For this review, take the finished solid that the model builds, in its own axes (mm). A direction names the side the tool comes from. Round coordinates to 2 decimals unless told otherwise and drop trailing zeros. Order: outer loops, then holes, each group sorted by start corner. A loop starts at its lowest first (then second) coordinate and runs counter-clockwise, first axis right, second up. Notation, with made-up numbers: (-40, 89.5) - (16, 89.5) arc R14 cw to (16, 101.5) - close; hole circle Ø4 at (53.25, 55). An arc over 180 degrees is marked (long way). One line per question, with ' | ' between items.
```python
from build123d import *

# Parameters (mm, degrees)
F0_W     = 480
F0_H     = 190
F1_DEPTH = 20
F2_W     = 500
F2_H     = 300
F3_DEPTH = 20
F4_W     = 10
F4_H     = 20
F4_W_2   = 500
F5_DEPTH = 170


# Not quite as in the source:
# - the program builds the solid bodies; features that only make, move or delete a surface that nothing else refers to are left out


with BuildPart() as f1:
    # F0 (on Top) → F1 (new body)
    with BuildSketch(Plane.XY):
        with Locations((10, -95)):
            Rectangle(F0_W, F0_H)
    extrude(amount=-F1_DEPTH)

    # F2 (on Front) → F3 (join)
    with BuildSketch(Plane.XZ):
        with Locations((0, -150)):
            Rectangle(F2_W, F2_H)
    extrude(amount=F3_DEPTH)

    # F4 (on face) → F5 (join)
    with BuildSketch(Plane.XZ.offset(20)):
        with Locations((255, -190)):
            Rectangle(F4_W, F4_H)
        with Locations((0, -190)):
            Rectangle(F4_W_2, F4_H)
    extrude(amount=F5_DEPTH)


solid = f1.part
```
(1) Insertion check: pin 1 (4 mm diameter, centred on x = 58.5, z = -208.5, fed in from -Y); pin 2 (12 mm diameter, centred on x = 165.5, y = -113, fed in from -Z); pin 3 (11 mm diameter, centred on x = 253.5, z = -191, fed in from +Y); pin 4 (10 mm diameter, centred on y = -101, z = -10, fed in from -X). Each pin has a flat end and moves straight along its axis. Give the tip position at first contact, or say it passes through.
Output values:
pin 1: y = -20 | pin 2: z = -200 | pin 3: y = 0 | pin 4: x = -230
(2) Mouldability with a two-part tool opening along Z and no side actions: class faces 1 (the flat face through (255, -20, -190)), 2 (the flat face through (-3, -94, 0)), 3 (the flat face through (-3, -20, -89)) as released by +Z, released by -Z, zero draft, split by the parting line, or undercut.
Output values:
face 1: zero draft | face 2: released by +Z | face 3: undercut
(3) For probe 1 along Z at (x, y) = (-85.5, -165); probe 2 along Y at (x, z) = (11, -23.5); probe 3 along X at (y, z) = (-19, -254.5), list the stretches that pass through material, from the lowest coordinate up. Write a range as [from, to].
Output values:
probe 1: [-200, -180], [-20, 0] | probe 2: [-20, 0] | probe 3: [-250, 250]
(4) For faces 4 (the flat face through (-230, -106, -10)), 5 (the flat face through (1, -104, -200)), 6 (the flat face through (7, -104, -20)), list the 3-axis set-ups (+Z, -Z, +X, -X, +Y, -Y) from which the entire face can be reached by the end or side of a thin tool; tool diameter is ignored.
Output values:
face 4: +Z, -X, -Y | face 5: -Z, +X, -X, -Y | face 6: +X, -X, -Y
(5) We need section A-A on y = -135. State the section outline as (x, z) points.
Output values:
outline: (-250, -200) - (260, -200) - (260, -180) - (-250, -180) - close; (-230, -20) - (250, -20) - (250, 0) - (-230, 0) - close
(6) We need section B-B on x = -56.5. State the section outline as (y, z) points, plus the area to 3 significant figures.
Output values:
outline: (-190, -200) - (-20, -200) - (-20, -300) - (0, -300) - (0, 0) - (-190, 0) - (-190, -20) - (-20, -20) - (-20, -180) - (-190, -180) - close | area: 12,800 mm^2
(7) We need section C-C on z = -151. State the section outline as (x, y) points.
Output values:
outline: (-250, -20) - (250, -20) - (250, 0) - (-250, 0) - close
